CAD build for the part. Positions are in the model's coordinates, mm. Face numbers are marked on the shaded views. A direction names the side the tool comes from. Give positions to 0.01 mm unless a question says otherwise; leave off trailing zeros. Order: outer loops, then holes, each group sorted by start corner. A loop starts at its lowest first (then second) coordinate and runs counter-clockwise, first axis right, second up.
Item 1: Wall check: L1, parallel to X at y = 6, z = -26.5 (3 decimals). Give the ranges that are in metal, low to high.
Item 2: Band-saw the part on A-A on y = 3. Give the cut face in (x, z) (3 decimals).
Item 3: Two-plate mould, pull along X, no slides. Class the marked faces 3, 4 and 5: released by +X, released by -X, zero draft, split by the parting line, or undercut.
Item 4: Flat gauge pins, fed straight in: P1, Ø3.5, axis at x = -18, y = -4.5, coming from the +Z side (3 decimals); P2, Ø8, axis at x = -12, y = 3, coming from the -Z side (3 decimals). Where does each tip first touch, or does it go through?
Item 5: Which spindle directions (+Z, -Z, +X, -X, +Y, -Y) get a long thin tool onto all of the face, cutting with end or side? Do the marked faces 1 and 2. Say none if no direction does.
Item 6: Band-saw the part on C-C on z = -48. Give the cut face in (x, y) (3 decimals), plus the area to 3 significant figures.
Item 7: Band-saw the part on B-B on x = 0.5. Give the cut face in (y, z) (3 decimals), plus the area to 3 significant figures.
Item 8: Band-saw the part on D-D on z = 58. Give the cut face in (x, y) (3 decimals), plus the area to 3 significant figures.
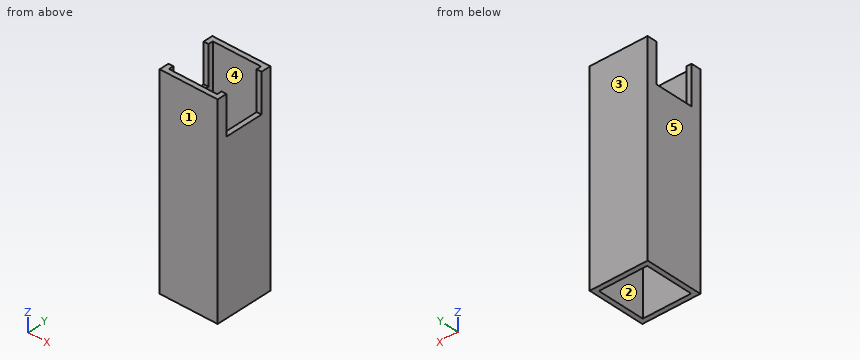
```python
from build123d import *

# Parameters (mm, degrees)
SKETCH1_W           = 38.1
SKETCH1_H           = 133.35
BOSS_EXTRUDE1_DEPTH = 19.05
SKETCH2_W           = 31.75
SKETCH2_H           = 31.75
CUT_EXTRUDE1_DEPTH  = 134.35
SKETCH3_W           = 25.4
SKETCH3_H           = 25.4
CUT_EXTRUDE2_DEPTH  = 39.1


with BuildPart() as part:
    # Sketch1 → Boss-Extrude1 (new body, symmetric)
    with BuildSketch(Plane(origin=(0, 0, 0), x_dir=(1, 0, 0), z_dir=(0, 1, 0))):
        Rectangle(SKETCH1_W, SKETCH1_H)
    extrude(amount=BOSS_EXTRUDE1_DEPTH, both=True)

    # Sketch2 → Cut-Extrude1 (cut, through all)
    with BuildSketch(Plane.XY.offset(66.675)):
        Rectangle(SKETCH2_W, SKETCH2_H)
    extrude(amount=-CUT_EXTRUDE1_DEPTH, mode=Mode.SUBTRACT)

    # Sketch3 → Cut-Extrude2 (cut, through all)
    with BuildSketch(Plane(origin=(19.05, 0, 0), x_dir=(0, 0, -1), z_dir=(1, 0, 0))):
        with Locations((-53.975, 0)):
            Rectangle(SKETCH3_W, SKETCH3_H)
    extrude(amount=-CUT_EXTRUDE2_DEPTH, mode=Mode.SUBTRACT)


solid = part.part
```
The answers:
1. L1: x = -19.05 to -15.875, 15.875 to 19.05
2. outline: (-19.05, -66.675) - (-15.875, -66.675) - (-15.875, 41.275) - (-19.05, 41.275) - close; (15.875, -66.675) - (19.05, -66.675) - (19.05, 41.275) - (15.875, 41.275) - close
3. face 3: zero draft
3. face 4: undercut
3. face 5: released by -X
4. P1: stops at z = 41.275
4. P2: stops at z = -66.675
5. face 1: +Z, -Z, +X, -X, -Y
5. face 2: +Z, -Z
6. outline: (-19.05, -19.05) - (19.05, -19.05) - (19.05, 19.05) - (-19.05, 19.05) - close; hole (-15.875, -15.875) - (15.875, -15.875) - (15.875, 15.875) - (-15.875, 15.875) - close
6. area: 444 mm2
7. outline: (-19.05, -66.675) - (-15.875, -66.675) - (-15.875, 66.675) - (-19.05, 66.675) - close; (15.875, -66.675) - (19.05, -66.675) - (19.05, 66.675) - (15.875, 66.675) - close
7. area: 847 mm2
8. outline: (-19.05, -19.05) - (19.05, -19.05) - (19.05, -12.7) - (15.875, -12.7) - (15.875, -15.875) - (-15.875, -15.875) - (-15.875, -12.7) - (-19.05, -12.7) - close; (-19.05, 12.7) - (-15.875, 12.7) - (-15.875, 15.875) - (15.875, 15.875) - (15.875, 12.7) - (19.05, 12.7) - (19.05, 19.05) - (-19.05, 19.05) - close
8. area: 282 mm2
